```python
from build123d import *

# Parameters (mm, degrees)
F2_W           = 73.3678117394
F2_H           = 19.5953426883
F3_DEPTH       = 47.4
F5_DEPTH       = 37.1
F6_R           = 11.2774131236
F7_DEPTH       = 16.7
F8_R           = 3.2
F9_DEPTH       = 36.8
F10_R          = 3.2661219018
F11_DEPTH      = 25
F12_R          = 3.175
F13_DEPTH      = 25
F13_DEPTH_BACK = 25


with BuildPart() as f1:
    # F0 (on Front) → F1 (revolve)
    with BuildSketch(Plane.XZ):
        with BuildLine():
            ThreePointArc((-23.3421701398, 7.9997662245), (-19.8064798686, 2.2157757205), (-14.8723184541, -2.4328480523))
            Line((-14.8723184541, -2.4328480523), (-14.8723184541, 8.0005478124))
            Line((-14.8723184541, 8.0005478124), (0, 8.0005478124))
            Line((0, 8.0005478124), (0, 43.8080292363))
            ThreePointArc((0, 43.8080292363), (-21.3722285148, 32.2277381458), (-23.3421701398, 7.9997662245))
        make_face()
        with BuildLine():
            ThreePointArc((-14.8723184541, -2.4328480523), (-7.8113091337, -5.9909309274), (0, -7.2161884465))
            Line((0, -7.2161884465), (0, 8.0005478124))
            Line((0, 8.0005478124), (-14.8723184541, 8.0005478124))
            Line((-14.8723184541, 8.0005478124), (-14.8723184541, -2.4328480523))
        make_face()
        with BuildLine():
            Line((-14.8723184541, -11.2020362965), (-14.8723184541, -30.4046204054))
            Line((-14.8723184541, -30.4046204054), (0, -30.4046204054))
            Line((0, -30.4046204054), (0, -7.2161884465))
            ThreePointArc((0, -7.2161884465), (-7.8113091337, -5.9909309274), (-14.8723184541, -2.4328480523))
            Line((-14.8723184541, -2.4328480523), (-14.8723184541, -11.2020362965))
        make_face()
        with BuildLine():
            Line((-23.3421701398, 7.9997662245), (-14.8723184541, -11.2020362965))
            Line((-14.8723184541, -11.2020362965), (-14.8723184541, -2.4328480523))
            ThreePointArc((-14.8723184541, -2.4328480523), (-19.8064798686, 2.2157757205), (-23.3421701398, 7.9997662245))
        make_face()
    revolve(axis=Axis((0, 0, 4.5623818878), (0, 0, -1)))

    # F2 (on Top) → F3 (cut, symmetric)
    with BuildSketch(Plane.XY):
        with Locations((-2.2661872208, 26.3196849264)):
            Rectangle(F2_W, F2_H)
        with Locations((-2.2661872208, -26.3196849264)):
            Rectangle(F2_W, F2_H)
    extrude(amount=F3_DEPTH, both=True, mode=Mode.SUBTRACT)

    # F4 (on Right) → F5 (cut, symmetric)
    with BuildSketch(Plane.YZ):
        with BuildLine():
            Line((9.3827452511, -5.8119617216), (9.3827452511, 45.4891547561))
            Line((9.3827452511, 45.4891547561), (0, 45.4891547561))
            Line((0, 45.4891547561), (0, -10.8119617216))
            Line((0, -10.8119617216), (4.3827452511, -10.8119617216))
            ThreePointArc((4.3827452511, -10.8119617216), (7.918279157, -9.3474956276), (9.3827452511, -5.8119617216))
        make_face()
        with BuildLine():
            Line((0, -10.8119617216), (0, 45.4891547561))
            Line((0, 45.4891547561), (-9.3827452511, 45.4891547561))
            Line((-9.3827452511, 45.4891547561), (-9.3827452511, -5.8119617216))
            ThreePointArc((-9.3827452511, -5.8119617216), (-7.918279157, -9.3474956276), (-4.3827452511, -10.8119617216))
            Line((-4.3827452511, -10.8119617216), (0, -10.8119617216))
        make_face()
    extrude(amount=F5_DEPTH, both=True, mode=Mode.SUBTRACT)

    # F6 (on face) → F7 (cut)
    with BuildSketch(Plane(origin=(0, 0, -30.4046204054), x_dir=(1, 0, 0), z_dir=(0, 0, -1))):
        Circle(F6_R)
    extrude(amount=-F7_DEPTH, mode=Mode.SUBTRACT)

    # F8 (on face) + F3_face1 (on face) → F9 (cut)
    with BuildSketch(Plane.XZ.offset(16.5220135823)):
        with Locations((0, 19.4492916284)):
            Circle(F8_R)
    with BuildSketch(Plane(origin=(0, 16.5220135823, 16.4645974536), x_dir=(-1, 0, 0), z_dir=(0, 1, 0))):
        with BuildLine():
            add(Edge.make_bspline(
                [(-16.488783279, -8.4648312291), (0, -34.870804714), (16.488783279, -8.4648312291)],
                knots=[-0.8799506859, -0.8799506859, -0.8799506859, 0.8799506859, 0.8799506859, 0.8799506859], degree=2, weights=[1, 1.4127920924, 1]))
            ThreePointArc((16.488783279, -8.4648312291), (0, 21.2707356053), (-16.488783279, -8.4648312291))
        make_face()
    extrude(amount=-F9_DEPTH, dir=(0, -1, 0), mode=Mode.SUBTRACT)

    # F10 (on face) → F11 (cut)
    with BuildSketch(Plane(origin=(0, 0, -13.7046204054), x_dir=(1, 0, 0), z_dir=(0, 0, -1))):
        Circle(F10_R)
    extrude(amount=-F11_DEPTH, mode=Mode.SUBTRACT)

    # F12 (on Right) → F13 (cut, two sides)
    with BuildSketch(Plane.YZ) as f13_sk:
        with Locations((0, -22.1496204054)):
            Circle(F12_R)
    extrude(amount=-F13_DEPTH, mode=Mode.SUBTRACT)
    extrude(f13_sk.sketch, amount=F13_DEPTH_BACK, mode=Mode.SUBTRACT)


solid = f1.part
```
Could you check a few things on this model? Use its own coordinates, in mm. A direction names the side the tool comes from. Round coordinates to 2 decimals unless told otherwise and drop trailing zeros. Loops run counter-clockwise (first coordinate to the right, second up) from the corner with the lowest first, then second, coordinate; pieces in that order, holes last.
Q1. Please list where these lines run through material, in increasing order: L1, parallel to Y at x = 14.5, z = 12; L2, parallel to X at y = 0, z = -12; L3, parallel to Z at x = 13.8, y = 0.
Q2. I want a section at B-B (x = 0). Give the number of separate pieces and of enclosed holes in the cut face, and give its area (3 significant figures).
Q3. I want a section at D-D (z = 24). Write out the boundary of the cut face in (x, y).
Q4. Thinking about a two-plate mould opening in Z: for faces 1 (the flat face through (11.1, 3.4, -30.405)), 2 (the cylindrical face through (-0.42, -13, 22.62)), 3 (the cylindrical face through (0.203, -7.957, -9.308)), which applies, pulls with the +Z half, pulls with the -Z half, needs draft (parallel to the pull), parting line crosses it, or undercut?
Q5. For P1, Ø7.5, axis at y = 0, z = -22.15, coming from the +X side; P2, Ø5, axis at x = -15, y = 13, coming from the +Z side; P3, Ø4, axis at y = 11.5, z = -21, coming from the -X side, each with a flat end and sliding along its axis, tell me the tip position at first contact or that it passes through.
Q6. I want a section at A-A (y = 0). Write out the boundary of the cut face in (x, z).
Q7. I want a section at C-C (z = -21). Write out the boundary of the cut face in (x, y).
Q8. On a 3-axis mill with a long thin cutter (end or side, diameter ignored), from which of +Z, -Z, +X, -X, +Y, -Y can I reach the whole of each face in a straight line? I mean faces 4 (the cylindrical face through (10.757, -3.387, -22.172)), 5 (the cylindrical face through (-0.71, 3.19, -12.28)), 6 (the flat face through (-5, 9.383, 18)). Say none if no direction works.
Answer below:
1. L1: y = -16.52 to -9.38, 9.38 to 16.52
1. L2: x = -14.87 to -3.27, 3.27 to 14.87
1. L3: z = -30.4 to -25.32, -18.97 to -10.81
2. separate pieces: 4
2. enclosed holes: 0
2. area: 829 mm2
3. outline: (-23.03, -9.38) arc R24.87 ccw to (-18.58, -16.52) - (18.58, -16.52) arc R24.87 ccw to (23.03, -9.38) - close; (-23.03, 9.38) - (23.03, 9.38) arc R24.87 ccw to (18.58, 16.52) - (-18.58, 16.52) arc R24.87 ccw to start
4. face 1: pulls with the -Z half
4. face 2: undercut
4. face 3: pulls with the +Z half
5. P1: stops at x = 14.87
5. P2: stops at z = 37
5. P3: stops at x = -11.44
6. outline: (-15.04, -10.81) - (-14.87, -11.2) - (-14.87, -18.97) - (-11.28, -18.97) - (-11.28, -13.7) - (-3.27, -13.7) - (-3.27, -10.81) - close; (-14.87, -30.4) - (-11.28, -30.4) - (-11.28, -25.32) - (-14.87, -25.32) - close; (3.27, -13.7) - (11.28, -13.7) - (11.28, -18.97) - (14.87, -18.97) - (14.87, -11.2) - (15.04, -10.81) - (3.27, -10.81) - close; (11.28, -30.4) - (14.87, -30.4) - (14.87, -25.32) - (11.28, -25.32) - close
7. outline: (-14.57, -2.96) arc R14.87 ccw to (14.57, -2.96) - (10.88, -2.96) arc R11.28 cw to (-10.88, -2.96) - close; (-14.57, 2.96) - (-10.88, 2.96) arc R11.28 cw to (10.88, 2.96) - (14.57, 2.96) arc R14.87 ccw to start
8. face 4: -Z
8. face 5: +Z, -Z
8. face 6: +Z, +X, -X
